Verification items for the finished model (mm, model axes). A direction names the side the tool comes from. Coordinates: 2 decimals unless noted, no trailing zeros. Loops run counter-clockwise (first coordinate to the right, second up) from the corner with the lowest first, then second, coordinate; pieces in that order, holes last.
Q1. Sectioned sample at B-B (y = -42). Enter the section's corners in (x, z), then the cut area to 3 significant figures.
Q2. Sectioned sample at D-D (y = -17.5). Enter the section's corners in (x, z), then the cut area to 3 significant figures.
Q3. Access from +Z, -Z, +X, -X, +Y, -Y to the whole of each face (thin tool, end or side, straight path). Record for faces 4 (the face through (-8, -51, 9.213)), 5 (the face through (0, -63.5, -11)).
Q4. Material ranges on probe 1 along Z at (x, y) = (4, -58); probe 2 along Y at (x, z) = (-4.5, 14); probe 3 along X at (y, z) = (-39, 14.5), recorded low to high.
Q5. Sectioned sample at C-C (x = 0). Enter the section's corners in (y, z).
Q6. Mould release check, pull along X, two halves, no side actions. Record for faces 1 (the face through (-5.506, -31.306, -24.796)), 2 (the face through (6.464, -51, 12)), 3 (the face through (0, 0, 0)): +X half, -X half, draft (parallel to the pull), parting line (faces both ways), or undercut.
Q7. Sectioned sample at A-A (z = 0). Enter the section's corners in (x, y), then the cut area to 3 significant figures.
Q8. Go/stop test with flat-tipped pins: P1, Ø11, axis at x = 0, y = -46, coming from the -Z side; P2, Ø1.5, axis at y = -56.5, z = 10, coming from the -X side; P3, Ø1.5, axis at y = -38.5, z = -15, coming from the -X side; P4, Ø5.5, axis at y = -46, z = -1, coming from the +X side. Record where each tip stops, or that it passes through.
```python
from build123d import *

# Parameters (mm, degrees)
F0_R     = 25.4
F1_DEPTH = 63.5
F2_W     = 19.278284
F2_H     = 18.425608
F3_DEPTH = 25.4
F4_W     = 13.516292
F4_H     = 9.261201
F5_DEPTH = 25.4


with BuildPart() as f1:
    # F0 (on Front) → F1 (new body)
    with BuildSketch(Plane.XZ):
        Circle(F0_R)
    extrude(amount=F1_DEPTH)

    # F2 (on face) → F3 (cut)
    with BuildSketch(Plane.XZ.offset(63.5)):
        Rectangle(F2_W, F2_H)
    extrude(amount=-F3_DEPTH, mode=Mode.SUBTRACT)

    # F4 (on face) → F5 (cut)
    with BuildSketch(Plane.XZ.offset(63.5)):
        with Locations((-0.294004, 10.932203)):
            Rectangle(F4_W, F4_H)
    extrude(amount=-F5_DEPTH, mode=Mode.SUBTRACT)


solid = f1.part
```
Geometry check:
1. outline: circle Ø50.8 at (0, 0); hole (-9.64, -9.21) - (9.64, -9.21) - (9.64, 9.21) - (6.46, 9.21) - (6.46, 15.56) - (-7.05, 15.56) - (-7.05, 9.21) - (-9.64, 9.21) - close
1. area: 1,590 mm2
2. outline: circle Ø50.8 at (0, 0)
2. area: 2,030 mm2
3. face 4: -Y
3. face 5: +Z, -Z, +X, -X, -Y
4. probe 1: z = -25.08 to -9.21, 15.56 to 25.08
4. probe 2: y = -38.1 to 0
4. probe 3: x = -20.85 to -7.05, 6.46 to 20.85
5. outline: (-63.5, -25.4) - (0, -25.4) - (0, 25.4) - (-63.5, 25.4) - (-63.5, 15.56) - (-38.1, 15.56) - (-38.1, -9.21) - (-63.5, -9.21) - close
6. face 1: parting line
6. face 2: undercut
6. face 3: draft
7. outline: (-25.4, -63.5) - (-9.64, -63.5) - (-9.64, -38.1) - (9.64, -38.1) - (9.64, -63.5) - (25.4, -63.5) - (25.4, 0) - (-25.4, 0) - close
7. area: 2,740 mm2
8. P1: stops at z = -25.4
8. P2: stops at x = -23.66
8. P3: stops at x = -21.03
8. P4: stops at x = 25.4
